Verification items for the finished model (mm, model axes). Coordinates: 2 decimals unless noted, no trailing zeros. Write each loop counter-clockwise with the first axis right and the second up, starting at its lowest first coordinate (ties: lowest second). Pieces come first, ordered by that corner, then holes. Notation, with made-up numbers: M 36.25,0.25 L 72.25,0.25 A10 cw 72.25,16.25 Z; hole C -5,49 d6. An arc over 180 degrees is marked long. Answer in a Markdown table with one row per item.
from build123d import *

# Parameters (mm, degrees)
SKETCH1_W           = 5
SKETCH1_H           = 100
SKETCH1_W_2         = 295
SKETCH1_H_2         = 150
BOSS_EXTRUDE1_DEPTH = 5
SKETCH2_W           = 70
SKETCH2_H           = 5
CUT_EXTRUDE1_DEPTH  = 5


with BuildPart() as part:
    # Sketch1 → Boss-Extrude1 (new body)
    with BuildSketch(Plane.XY):
        with Locations((-297.5, 75)):
            Rectangle(SKETCH1_W, SKETCH1_H)
        with Locations((-147.5, 75)):
            Rectangle(SKETCH1_W_2, SKETCH1_H_2)
        with Locations((2.5, 75)):
            Rectangle(SKETCH1_W, SKETCH1_H)
    extrude(amount=BOSS_EXTRUDE1_DEPTH)

    # Sketch2 → Cut-Extrude1 (cut)
    with BuildSketch(Plane.XY.offset(5)):
        with Locations((-210, 7.5)):
            Rectangle(SKETCH2_W, SKETCH2_H)
        with Locations((-85, 7.5)):
            Rectangle(SKETCH2_W, SKETCH2_H)
    extrude(amount=-CUT_EXTRUDE1_DEPTH, mode=Mode.SUBTRACT)


solid = part.part
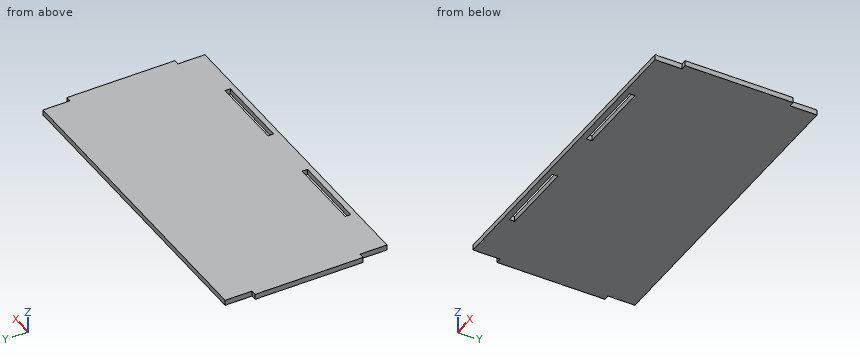
1) Depth check by flat-ended pin: pin 1 (1.5 mm diameter, centred on y = 138, z = 3, fed in from +X); pin 2 (1.5 mm diameter, centred on y = 8.5, z = 1.5, fed in from -X); pin 3 (2.5 mm diameter, centred on x = 1.5, z = 2, fed in from -Y). Enter the tip coordinate at first touch or a pass-through.
Response values:
| item | result |
|---|---|
| pin 1 | stops at x = 0 |
| pin 2 | stops at x = -295 |
| pin 3 | stops at y = 25 |
2) Sectioned sample at B-B (z = 3.75). Record the cut outline in (x, y), then the cut area to 4 significant figures.
Response values:
| item | result |
|---|---|
| outline | M -300,25 L -295,25 L -295,0 L 0,0 L 0,25 L 5,25 L 5,125 L 0,125 L 0,150 L -295,150 L -295,125 L -300,125 Z; hole M -245,5 L -175,5 L -175,10 L -245,10 Z; hole M -120,5 L -50,5 L -50,10 L -120,10 Z |
| area | 44,550 mm² |
3) Sectioned sample at A-A (x = -188). Record the cut outline in (y, z).
Response values:
| item | result |
|---|---|
| outline | M 0,0 L 5,0 L 5,5 L 0,5 Z; M 10,0 L 150,0 L 150,5 L 10,5 Z |
4) Thickness scan on L1, parallel to Y at x = -216.5, z = 4.35; L2, parallel to X at y = 14, z = 1.85. Record the ranges inside material, lowest first. Write a range as [from, to].
Response values:
| item | result |
|---|---|
| L1 | y = [0, 5], [10, 150] |
| L2 | x = [-295, 0] |
